Model file for the job. Use its own axes, mm. Round coordinates to 2 decimals unless told otherwise and drop trailing zeros. Loops run counter-clockwise (first coordinate to the right, second up) from the corner with the lowest first, then second, coordinate; pieces in that order, holes last. Notation, with made-up numbers: (48, 55.25) -> (53, 55.25) arc R22 cw to (53, 90.25) -> close; hole circle Ø2 at (-1.75, 40.5). An arc over 180 degrees is marked (long way). Use a Markdown table: item, result. Add a question column.
```python
from build123d import *

# Parameters (mm, degrees)
SCALE1_START       = 1.378692074
SCALE1_OUTLINE_R   = 0.4392
SCALE1_DEPTH       = 0.244
CUT_EXTRUDE1_DEPTH = 2.54
CUT_EXTRUDE2_DEPTH = 51.110559093
CUT_EXTRUDE3_DEPTH = 51.110559093
CUT_EXTRUDE4_DEPTH = 51.110559093


with BuildPart() as part:
    # Scale1: read off the stored shape, not the designer's step
    # Scale1 outline → Scale1 (new body)
    with BuildSketch(Plane.XY.offset(SCALE1_START)):
        with BuildLine():
            Line((17.68301566, 43.704577473), (17.346177673, 41.830755017))
            ThreePointArc((17.346177673, 41.830755017), (17.037161165, 41.420736581), (16.523766226, 41.426389643))
            ThreePointArc((16.523766226, 41.426389643), (13.552700425, 42.459086685), (10.410542545, 42.602401154))
            ThreePointArc((10.410542545, 42.602401154), (9.854263516, 42.795493333), (9.640942513, 43.344333108))
            ThreePointArc((9.640942513, 43.344333108), (9.437328912, 43.59391361), (9.172716599, 43.410258363))
            ThreePointArc((9.172716599, 43.410258363), (8.792265037, 43.128007225), (8.459444481, 43.465111917))
            ThreePointArc((8.459444481, 43.465111917), (8.269075619, 43.807602921), (7.883340454, 43.876514268))
            ThreePointArc((7.883340454, 43.876514268), (7.526718951, 44.047734987), (7.645582772, 44.425050271))
            ThreePointArc((7.645582772, 44.425050271), (7.724200076, 45.050111764), (7.096911805, 44.991871103))
            ThreePointArc((7.096911805, 44.991871103), (6.923054486, 44.682724324), (6.79514349, 44.351911876))
            Line((6.79514349, 44.351911876), (6.650098626, 43.450480425))
            ThreePointArc((6.650098626, 43.450480425), (6.721898103, 42.933324679), (7.071222107, 42.545280904))
            ThreePointArc((7.071222107, 42.545280904), (8.30836308, 42.068484056), (9.633857836, 42.038207468))
            ThreePointArc((9.633857836, 42.038207468), (13.079663737, 42.019930147), (16.355693709, 40.951501394))
            ThreePointArc((16.355693709, 40.951501394), (16.569606698, 40.488798349), (16.169670974, 40.172721944))
            Line((16.169670974, 40.172721944), (12.996206362, 40.526319917))
            ThreePointArc((12.996206362, 40.526319917), (11.358592721, 39.478912268), (12.040129402, 37.658376915))
            ThreePointArc((12.040129402, 37.658376915), (13.31395276, 36.623381651), (14.225764982, 35.258669367))
            ThreePointArc((14.225764982, 35.258669367), (14.386229966, 34.744015637), (14.401396414, 34.205139535))
            ThreePointArc((14.401396414, 34.205139535), (14.672806749, 33.376647317), (15.474699865, 33.034550319))
            Line((15.474699865, 33.034550319), (17.348101609, 33.034550317))
            ThreePointArc((17.348101609, 33.034550317), (18.244587572, 32.671085647), (18.634843629, 31.785933762))
            ThreePointArc((18.634843629, 31.785933762), (19.451177789, 31.997778319), (19.942322167, 32.683385187))
            Line((19.942322167, 32.683385187), (21.269314636, 37.404760613))
            ThreePointArc((21.269314636, 37.404760613), (21.73439895, 38.387008616), (22.497682404, 39.16064479))
            Line((22.497682404, 39.16064479), (23.128103851, 39.765569271))
            ThreePointArc((23.128103851, 39.765569271), (23.52490002, 40.486669007), (23.253920075, 41.263844598))
            Line((23.253920075, 41.263844598), (22.452558823, 42.115876451))
            ThreePointArc((22.452558823, 42.115876451), (22.115289154, 42.23834678), (21.816559174, 42.039575025))
            Line((21.816559174, 42.039575025), (21.688661164, 41.814089241))
            Line((21.688661164, 41.814089241), (21.575749212, 41.910847183))
            ThreePointArc((21.575749212, 41.910847183), (20.868513286, 41.926668482), (20.744543825, 42.623134233))
            Line((20.744543825, 42.623134233), (18.940412338, 44.169153428))
            ThreePointArc((18.940412338, 44.169153428), (18.175234277, 44.306254238), (17.68301566, 43.704577473))
        make_face()
        with Locations((15.322718522, 36.789890957)):
            Circle(SCALE1_OUTLINE_R, mode=Mode.SUBTRACT)
        with Locations((12.792357561, 39.068616569)):
            Circle(SCALE1_OUTLINE_R, mode=Mode.SUBTRACT)
    extrude(amount=SCALE1_DEPTH)

    # Scale1 2 outline → Scale1 2 (revolve, cut)
    with BuildSketch(Plane(origin=(18.426504279, 37.473794578, 0), x_dir=(1, 0, 0), z_dir=(0, -1, 0))):
        Polygon((0, 1.378692074), (0.732, 1.378692074), (0.488, 1.622692074), (0, 1.622692074), align=None)
    revolve(axis=Axis((18.426504279, 37.473794578, 0), (0, 0, 1)), mode=Mode.SUBTRACT)

    # Sketch1 → Cut-Extrude1 (cut)
    with BuildSketch(Plane(origin=(0, 0, 1.378692074), x_dir=(-1, 0, 0), z_dir=(0, 0, -1))):
        with BuildLine():
            Line((-21.688661166, 41.81408924), (-21.982980789, 42.999564373))
            Line((-21.982980789, 42.999564373), (-25.421126936, 39.405059446))
            Line((-25.421126936, 39.405059446), (-20.605818398, 35.044072901))
            add(Edge.make_bspline(
                [(-21.688661166, 41.81408924), (-19.489266143, 39.961862231), (-18.997440369, 38.289314262), (-20.605818398, 35.044072901)],
                knots=[0, 0, 0, 0, 1, 1, 1, 1], degree=3))
        make_face()
    extrude(amount=-CUT_EXTRUDE1_DEPTH, mode=Mode.SUBTRACT)

    # Sketch2 → Cut-Extrude2 (cut, through all)
    with BuildSketch(Plane(origin=(0, 0, 1.378692074), x_dir=(-1, 0, 0), z_dir=(0, 0, -1))):
        with BuildLine():
            Line((-17.348101609, 33.534550318), (-15.46825055, 33.534550318))
            ThreePointArc((-15.46825055, 33.534550318), (-15.042927497, 33.712833322), (-14.89843377, 34.150790045))
            ThreePointArc((-14.89843377, 34.150790045), (-14.879423654, 34.826234772), (-14.678291655, 35.471318396))
            ThreePointArc((-14.678291655, 35.471318396), (-14.660582055, 35.508670476), (-14.642615597, 35.545899689))
            ThreePointArc((-14.642615597, 35.545899689), (-14.616480362, 35.726837837), (-14.700216201, 35.889349293))
            Line((-14.700216201, 35.889349293), (-14.751462797, 35.940595889))
            ThreePointArc((-14.751462797, 35.940595889), (-14.895326012, 36.020592881), (-15.059742801, 36.012639096))
            ThreePointArc((-15.059742801, 36.012639096), (-15.580994431, 36.011064763), (-15.998016925, 36.323791449))
            ThreePointArc((-15.998016925, 36.323791449), (-16.074795707, 36.400479379), (-16.173833875, 36.44483545))
            Line((-16.173833875, 36.44483545), (-17.161803556, 36.685788167))
            ThreePointArc((-17.161803556, 36.685788167), (-17.321020312, 36.681092865), (-17.455391032, 36.595556142))
            ThreePointArc((-17.455391032, 36.595556142), (-18.245306435, 36.177055965), (-19.119682785, 36.362998806))
            ThreePointArc((-19.119682785, 36.362998806), (-19.377471249, 36.391695847), (-19.561279678, 36.208685263))
            Line((-19.561279678, 36.208685263), (-20.072904791, 34.995897621))
            Line((-20.072904791, 34.995897621), (-19.460972938, 32.818673477))
            ThreePointArc((-19.460972938, 32.818673477), (-19.437288786, 32.748237282), (-19.40663946, 32.680540786))
            ThreePointArc((-19.40663946, 32.680540786), (-19.149382906, 32.518029269), (-18.882393628, 32.66400068))
            ThreePointArc((-18.882393628, 32.66400068), (-18.230131749, 33.301751954), (-17.348101609, 33.534550318))
        make_face()
    extrude(amount=-CUT_EXTRUDE2_DEPTH, mode=Mode.SUBTRACT)

    # Sketch3 → Cut-Extrude3 (cut, through all)
    with BuildSketch(Plane(origin=(0, 0, 1.378692074), x_dir=(-1, 0, 0), z_dir=(0, 0, -1))):
        with BuildLine():
            Line((-20.496817758, 41.658030449), (-17.346177676, 41.830755017))
            Line((-17.346177676, 41.830755017), (-17.346177676, 45.415633963))
            Line((-17.346177676, 45.415633963), (-20.923893138, 43.312384261))
            ThreePointArc((-20.923893138, 43.312384261), (-20.253979171, 42.603021979), (-20.496817758, 41.658030449))
        make_face()
    extrude(amount=-CUT_EXTRUDE3_DEPTH, mode=Mode.SUBTRACT)

    # Sketch4 → Cut-Extrude4 (cut, through all)
    with BuildSketch(Plane(origin=(0, 0, 1.378692074), x_dir=(-1, 0, 0), z_dir=(0, 0, -1))):
        with BuildLine():
            Line((-17.455852383, 40.574313146), (-18.8042073, 40.524397539))
            ThreePointArc((-18.8042073, 40.524397539), (-19.040601602, 40.394153532), (-19.076676041, 40.126675679))
            Line((-19.076676041, 40.126675679), (-18.682397479, 38.984966524))
            ThreePointArc((-18.682397479, 38.984966524), (-18.575024983, 38.840086232), (-18.403989188, 38.782938099))
            ThreePointArc((-18.403989188, 38.782938099), (-17.597035683, 38.48688171), (-17.14755053, 37.754224599))
            ThreePointArc((-17.14755053, 37.754224599), (-17.069108072, 37.608838613), (-16.925594615, 37.527020573))
            Line((-16.925594615, 37.527020573), (-16.148609211, 37.337524127))
            ThreePointArc((-16.148609211, 37.337524127), (-16.00427201, 37.33806247), (-15.876892057, 37.405943726))
            ThreePointArc((-15.876892057, 37.405943726), (-15.557022892, 37.584705893), (-15.191334883, 37.60803988))
            ThreePointArc((-15.191334883, 37.60803988), (-15.051369663, 37.618828593), (-14.931636329, 37.692112887))
            Line((-14.931636329, 37.692112887), (-14.130011628, 38.493737588))
            ThreePointArc((-14.130011628, 38.493737588), (-14.053640182, 38.623615493), (-14.050038507, 38.774240511))
            ThreePointArc((-14.050038507, 38.774240511), (-14.083791972, 39.093431642), (-14.037801355, 39.411090481))
            ThreePointArc((-14.037801355, 39.411090481), (-14.100156714, 39.686879536), (-14.364076124, 39.788340557))
            Line((-14.364076124, 39.788340557), (-16.044195491, 39.579464149))
            ThreePointArc((-16.044195491, 39.579464149), (-16.744622059, 39.75112655), (-17.15323559, 40.345349015))
            ThreePointArc((-17.15323559, 40.345349015), (-17.263742997, 40.513756841), (-17.455852383, 40.574313146))
        make_face()
    extrude(amount=-CUT_EXTRUDE4_DEPTH, mode=Mode.SUBTRACT)


solid = part.part
```
1) Cut at A-A on x = 11.5. Write the cut outline in (y, z).
2) Cut at B-B on y = 34.5. Write the cut outline in (x, z).
3) Wall check: probe 1 along Y at (x, z) = (15, 1.5); probe 2 along X at (y, z) = (37, 1.5); probe 3 along Y at (x, z) = (17.25, 1.5). Give the ranges that are in metal, low to high. Write a range as from..to.
4) Pin check, flat tip, straight feed: pin 1 Ø8 at (x, y) = (9, 39) entering from +Z. Stop position of the tip, or through.
5) Cut at D-D on x = 8.75. Write the cut outline in (y, z), and give its area (3 significant figures).
6) Cut at C-C on z = 1.55. Count the separate pieces of the cut face and the enclosed holes in it, and give its area (3 significant figures).
Established:
| question | item | result |
|---|---|---|
| 1 | outline | (38.19, 1.38) -> (39.79, 1.38) -> (39.79, 1.62) -> (38.19, 1.62) -> close; (42.16, 1.38) -> (42.66, 1.38) -> (42.66, 1.62) -> (42.16, 1.62) -> close |
| 2 | outline | (14.41, 1.38) -> (14.91, 1.38) -> (14.91, 1.62) -> (14.41, 1.62) -> close; (19.93, 1.38) -> (20.45, 1.38) -> (20.45, 1.62) -> (19.93, 1.62) -> close |
| 3 | probe 1 | y = 33.14..33.77, 36.03..36.49, 37.09..37.64, 39.71..40.3, 41.53..42.08 |
| 3 | probe 2 | x = 12.94..14.94, 15.71..18.04, 18.81..19.84 |
| 3 | probe 3 | y = 33.03..33.53, 36.69..38.05, 40.5..41.6 |
| 4 | pin 1 | stops at z = 1.62 |
| 5 | outline | (42.01, 1.38) -> (43.13, 1.38) -> (43.13, 1.62) -> (42.01, 1.62) -> close |
| 5 | area | 0.275 mm^2 |
| 6 | separate pieces | 1 |
| 6 | enclosed holes | 5 |
| 6 | area | 41.9 mm^2 |
